The model under review builds one solid part; all positions refer to its coordinate system, in mm. Face numbers are marked on the shaded views. A direction names the side the tool comes from. Round coordinates to 2 decimals unless told otherwise and drop trailing zeros. Order: outer loops, then holes, each group sorted by start corner. A loop starts at its lowest first (then second) coordinate and runs counter-clockwise, first axis right, second up.
1) Clearance check with flat-ended pins moving along their axes: P1, Ø1, axis at x = 39.5, z = -15, coming from the -Y side; P2, Ø6, axis at x = 101, y = 7, coming from the -Z side; P3, Ø8, axis at x = 114.5, y = 10.5, coming from the +Z side. State where each tip first meets the part, or that it passes through.
2) Machinability: for the marked faces 1, 2, 3, 4 and 5, which of the approach directions +Z, -Z, +X, -X, +Y, -Y give a long, thin tool a straight path to every point of the face, cutting with its end or side? Answer none if there is none.
3) Consider section C-C (x = 110). Give the boundary of the cut face in (y, z).
4) Mouldability with a two-part tool opening along X and no side actions: class the marked faces 6, 7, 8 and 9 as pulls with the +X half, pulls with the -X half, needs draft (parallel to the pull), parting line crosses it, or undercut.
5) Consider section B-B (z = -41). Give the boundary of the cut face in (x, y), then the cut area to 3 significant figures.
6) To check wall thickness, follow L1, parallel to X at y = 14, z = 38; L2, parallel to Z at x = 127.5, y = 1; L3, parallel to X at y = 16.5, z = -19.5. State the ranges of each line that lie inside material, in increasing order.
from build123d import *

# Parameters (mm, degrees)
CORNERBOSS_EXTRUDE1_DEPTH               = 20
SHELL1_T                                = -3
PADSKETCH2_R                            = 12
PADSKETCH2_R_2                          = 5
PADBOSS_EXTRUDE2_DEPTH                  = 10
STEPPERRODHOLESKETCH3_R                 = 5.1
STEPPERRODHOLESKETCH3_R_2               = 2
STEPPERRODHOLECUT_EXTRUDE1_DEPTH        = 255.298998474
THREADEDNUTMOUNTHOLESSKETCH4_R          = 2
THREADEDNUTMOUNTHOLESCUT_EXTRUDE2_DEPTH = 10
TLPEGHOLESKETCH1_W                      = 10
TLPEGHOLESKETCH1_H                      = 14
TLPEGHOLECUT_EXTRUDE1_DEPTH             = 3
BOTTOMPEGSKETCH2_W                      = 9.8
BOTTOMPEGSKETCH2_H                      = 13.9
BOTTOMPEGBOSS_EXTRUDE1_DEPTH            = 3.1
BOTTOMPEGCAPSKETCH3_W                   = 16
BOTTOMPEGCAPSKETCH3_H                   = 17
BOTTOMPEGCAPBOSS_EXTRUDE2_DEPTH         = 3
BEDCENTERHOLECUTSKETCH1_W               = 10
BEDCENTERHOLECUTSKETCH1_H               = 14
BEDCENTERHOLECUT_EXTRUDE1_DEPTH         = 3


with BuildPart() as part:
    # CornerSketch1 → CornerBoss-Extrude1 (new body)
    with BuildSketch(Plane(origin=(0, 0, 0), x_dir=(1, 0, 0), z_dir=(0, 1, 0))):
        with BuildLine():
            Line((210, -70), (140, -70))
            Line((140, -70), (140, 0))
            Line((140, 0), (0, 0))
            Line((0, 0), (0, 80))
            Line((0, 80), (176, 80))
            Line((176, 80), (176, 125.825))
            ThreePointArc((176, 125.825), (193, 142.825), (210, 125.825))
            Line((210, 125.825), (210, -70))
        make_face()
    extrude(amount=CORNERBOSS_EXTRUDE1_DEPTH)

    # Shell1
    shell1_openings = [part.faces().sort_by_distance(p)[0] for p in [
        (126.932214483, 0, -30.416556174),
    ]]
    offset(amount=SHELL1_T, openings=shell1_openings, kind=Kind.INTERSECTION)

    # PadSketch2 → PadBoss-Extrude2 (add)
    with BuildSketch(Plane.XZ.offset(-17)):
        with Locations(Location((193, -125.825, 0), (0, 0, 90))):
            Circle(PADSKETCH2_R)
        with Locations(Location((169, -63, 0), (0, 0, 90))):
            Circle(PADSKETCH2_R_2)
    extrude(amount=PADBOSS_EXTRUDE2_DEPTH)

    # StepperRodHoleSketch3 → StepperRodHoleCut-Extrude1 (cut, through all)
    with BuildSketch(Plane.XZ.offset(-7)):
        with Locations(Location((193, -125.825, 0), (0, 0, 270))):
            Circle(STEPPERRODHOLESKETCH3_R)
        with Locations(Location((169, -63, 0), (0, 0, 270))):
            Circle(STEPPERRODHOLESKETCH3_R_2)
    extrude(amount=-STEPPERRODHOLECUT_EXTRUDE1_DEPTH, mode=Mode.SUBTRACT)

    # ThreadedNutMountHolesSketch4 → ThreadedNutMountHolesCut-Extrude2 (cut)
    with BuildSketch(Plane(origin=(0, 7, 0), x_dir=(-1, 0, 0), z_dir=(0, -1, 0))):
        with Locations(Location((-193, 133.825, 0), (0, 0, 90))):
            Circle(THREADEDNUTMOUNTHOLESSKETCH4_R)
        with Locations(Location((-185, 125.825, 0), (0, 0, 90))):
            Circle(THREADEDNUTMOUNTHOLESSKETCH4_R)
        with Locations(Location((-201, 125.825, 0), (0, 0, 90))):
            Circle(THREADEDNUTMOUNTHOLESSKETCH4_R)
        with Locations(Location((-193, 117.825, 0), (0, 0, 90))):
            Circle(THREADEDNUTMOUNTHOLESSKETCH4_R)
    extrude(amount=-THREADEDNUTMOUNTHOLESCUT_EXTRUDE2_DEPTH, mode=Mode.SUBTRACT)

    # TLPegHoleSketch1 → TLPegHoleCut-Extrude1 (cut)
    with BuildSketch(Plane.ZY):
        with Locations((-65, 7)):
            Rectangle(TLPEGHOLESKETCH1_W, TLPEGHOLESKETCH1_H)
    extrude(amount=-TLPEGHOLECUT_EXTRUDE1_DEPTH, mode=Mode.SUBTRACT)

    # BottomPegSketch2 → BottomPegBoss-Extrude1 (add)
    with BuildSketch(Plane.XY.offset(70)):
        with Locations((195, 6.95)):
            Rectangle(BOTTOMPEGSKETCH2_W, BOTTOMPEGSKETCH2_H)
    extrude(amount=BOTTOMPEGBOSS_EXTRUDE1_DEPTH)

    # BottomPegCapSketch3 → BottomPegCapBoss-Extrude2 (add)
    with BuildSketch(Plane.XY.offset(73.1)):
        with Locations((195.1, 8.5)):
            Rectangle(BOTTOMPEGCAPSKETCH3_W, BOTTOMPEGCAPSKETCH3_H)
    extrude(amount=BOTTOMPEGCAPBOSS_EXTRUDE2_DEPTH)

    # BedCenterHoleCutSketch1 → BedCenterHoleCut-Extrude1 (cut)
    with BuildSketch(Plane.XY):
        with Locations((35, 7)):
            Rectangle(BEDCENTERHOLECUTSKETCH1_W, BEDCENTERHOLECUTSKETCH1_H)
    extrude(amount=-BEDCENTERHOLECUT_EXTRUDE1_DEPTH, mode=Mode.SUBTRACT)


solid = part.part
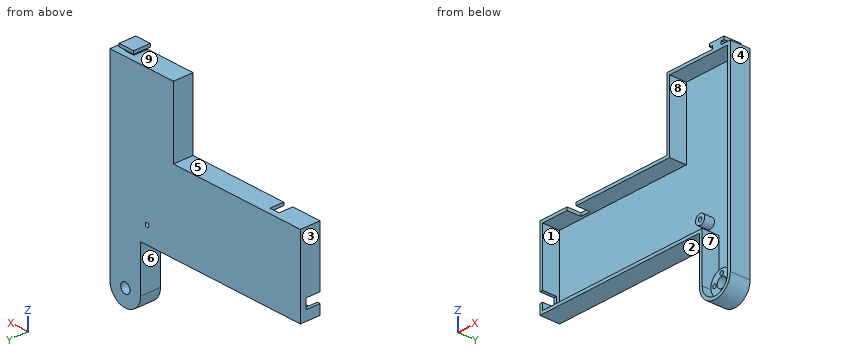
Answer below:
1. P1: stops at y = 17
1. P2: stops at z = -80
1. P3: stops at z = 0
2. face 1: -Y
2. face 2: -Z, -X, +Y, -Y
2. face 3: +Z, -Z, -X, +Y, -Y
2. face 4: +Z, -Z, +X, +Y, -Y
2. face 5: +Z, -X, +Y, -Y
3. outline: (0, -80) - (20, -80) - (20, 0) - (0, 0) - (0, -3) - (17, -3) - (17, -77) - (0, -77) - close
4. face 6: pulls with the -X half
4. face 7: undercut
4. face 8: undercut
4. face 9: needs draft
5. outline: (0, 0) - (3, 0) - (3, 17) - (207, 17) - (207, 0) - (210, 0) - (210, 20) - (0, 20) - close
5. area: 732 mm2
6. L1: x = 140 to 143, 207 to 210
6. L2: z = -80 to -77, -3 to 0
6. L3: x = 0 to 3, 207 to 210
